The model under review builds one solid part; all positions refer to its coordinate system, in mm. Face numbers are marked on the shaded views. A direction names the side the tool comes from. Give positions to 0.01 mm unless a question says otherwise; leave off trailing zeros. Order: outer loops, then holes, each group sorted by start corner. A loop starts at its lowest first (then second) coordinate and runs counter-clockwise, first axis right, second up. Notation, with made-up numbers: (41, 16) - (80, 16) arc R21 ccw to (80, 52) - close; hole circle Ø6 at (-38.5, -23.5). An arc over 180 degrees is marked (long way). Use CSV: the item, a comma, the result in double quotes. Start each with the question number.
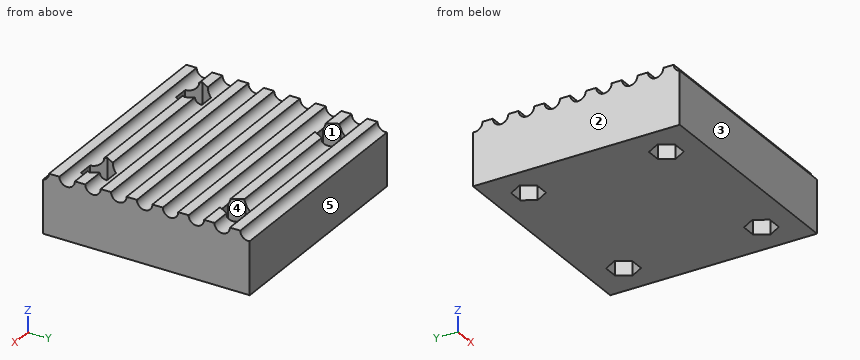
```python
from build123d import *

# Parameters (mm, degrees)
SKETCH3_W           = 26
SKETCH3_H           = 24
BOSS_EXTRUDE2_DEPTH = 7
SKETCH7_R           = 0.9
CUT_EXTRUDE1_DEPTH  = 27


with BuildPart() as part:
    # Sketch3 → Boss-Extrude2 (new body)
    with BuildSketch(Plane.XY):
        with Locations((13, 12)):
            Rectangle(SKETCH3_W, SKETCH3_H)
        Polygon((5.732050808, 4), (4.866025404, 5.5), (3.133974596, 5.5), (2.267949192, 4), (3.133974596, 2.5), (4.866025404, 2.5), align=None, mode=Mode.SUBTRACT)
        Polygon((5.732050808, 20), (4.866025404, 21.5), (3.133974596, 21.5), (2.267949192, 20), (3.133974596, 18.5), (4.866025404, 18.5), align=None, mode=Mode.SUBTRACT)
        Polygon((23.732050808, 20), (22.866025404, 21.5), (21.133974596, 21.5), (20.267949192, 20), (21.133974596, 18.5), (22.866025404, 18.5), align=None, mode=Mode.SUBTRACT)
        Polygon((23.732050808, 4), (22.866025404, 5.5), (21.133974596, 5.5), (20.267949192, 4), (21.133974596, 2.5), (22.866025404, 2.5), align=None, mode=Mode.SUBTRACT)
    extrude(amount=BOSS_EXTRUDE2_DEPTH)

    # Sketch7 → Cut-Extrude1 (cut, through all)
    with BuildSketch(Plane(origin=(26, 0, 0), x_dir=(0, 0, -1), z_dir=(1, 0, 0))):
        with Locations((-7, 23.8)):
            Circle(SKETCH7_R)
        with Locations((-7, 20.8)):
            Circle(SKETCH7_R)
        with Locations((-7, 17.8)):
            Circle(SKETCH7_R)
        with Locations((-7, 14.8)):
            Circle(SKETCH7_R)
        with Locations((-7, 11.8)):
            Circle(SKETCH7_R)
        with Locations((-7, 8.8)):
            Circle(SKETCH7_R)
        with Locations((-7, 5.8)):
            Circle(SKETCH7_R)
        with Locations((-7, 2.8)):
            Circle(SKETCH7_R)
        with Locations((-7, -0.2)):
            Circle(SKETCH7_R)
    extrude(amount=-CUT_EXTRUDE1_DEPTH, mode=Mode.SUBTRACT)


solid = part.part
```
1. Consider section D-D (y = 2.8). Give the boundary of the cut face in (x, z).
2. Consider section A-A (x = 3.5). Give the boundary of the cut face in (y, z).
3. Consider section B-B (z = 3.5). Give the boundary of the cut face in (x, y), and give its area (3 significant figures).
4. Tool access review of the marked faces 4 and 5: name each direction out of +Z, -Z, +X, -X, +Y, -Y from which nothing blocks a thin tool from reaching the whole face with its end or side.
5. Consider section C-C (x = 18). Give the boundary of the cut face in (y, z), and give its area (3 significant figures).
6. To check wall thickness, follow L1, parallel to Y at x = 3.5, z = 2; L2, parallel to Y at x = 23.5, z = 0.5; L3, parallel to Z at x = 16.5, y = 15.5. State the ranges of each line that lie inside material, in increasing order. Write a range as [from, to].
7. Mouldability with a two-part tool opening along X and no side actions: class the marked faces 1, 2 and 3 as pulls with the +X half, pulls with the -X half, needs draft (parallel to the pull), parting line crosses it, or undercut.
Answers follow:
1,outline,"(0, 0) - (2.96, 0) - (2.96, 6.1) - (0, 6.1) - close; (5.04, 0) - (20.96, 0) - (20.96, 6.1) - (5.04, 6.1) - close; (23.04, 0) - (26, 0) - (26, 6.1) - (23.04, 6.1) - close"
2,outline,"(0, 0) - (2.5, 0) - (2.5, 6.15) arc R0.9 cw to (1.9, 7) - (0.7, 7) arc R0.9 cw to (0, 6.12) - close; (5.5, 0) - (18.5, 0) - (18.5, 6.43) arc R0.9 cw to (16.9, 7) - (15.7, 7) arc R0.9 cw to (13.9, 7) - (12.7, 7) arc R0.9 cw to (10.9, 7) - (9.7, 7) arc R0.9 cw to (7.9, 7) - (6.7, 7) arc R0.9 cw to (5.5, 6.15) - close; (21.5, 0) - (24, 0) - (24, 6.12) arc R0.9 cw to (22.9, 7) - (21.7, 7) arc R0.9 cw to (21.5, 6.43) - close"
3,outline,"(0, 0) - (26, 0) - (26, 24) - (0, 24) - close; hole (2.27, 4) - (3.13, 2.5) - (4.87, 2.5) - (5.73, 4) - (4.87, 5.5) - (3.13, 5.5) - close; hole (2.27, 20) - (3.13, 18.5) - (4.87, 18.5) - (5.73, 20) - (4.87, 21.5) - (3.13, 21.5) - close; hole (20.27, 4) - (21.13, 2.5) - (22.87, 2.5) - (23.73, 4) - (22.87, 5.5) - (21.13, 5.5) - close; hole (20.27, 20) - (21.13, 18.5) - (22.87, 18.5) - (23.73, 20) - (22.87, 21.5) - (21.13, 21.5) - close"
3,area,"593 mm^2"
4,face 4,"+Z, -Z"
4,face 5,"+Z, -Z, +X, -X, +Y"
5,outline,"(0, 0) - (24, 0) - (24, 6.12) arc R0.9 cw to (22.9, 7) - (21.7, 7) arc R0.9 cw to (19.9, 7) - (18.7, 7) arc R0.9 cw to (16.9, 7) - (15.7, 7) arc R0.9 cw to (13.9, 7) - (12.7, 7) arc R0.9 cw to (10.9, 7) - (9.7, 7) arc R0.9 cw to (7.9, 7) - (6.7, 7) arc R0.9 cw to (4.9, 7) - (3.7, 7) arc R0.9 cw to (1.9, 7) - (0.7, 7) arc R0.9 cw to (0, 6.12) - close"
5,area,"158 mm^2"
6,L1,"y = [0, 2.5], [5.5, 18.5], [21.5, 24]"
6,L2,"y = [0, 3.6], [4.4, 19.6], [20.4, 24]"
6,L3,"z = [0, 6.43]"
7,face 1,"undercut"
7,face 2,"pulls with the -X half"
7,face 3,"needs draft"
